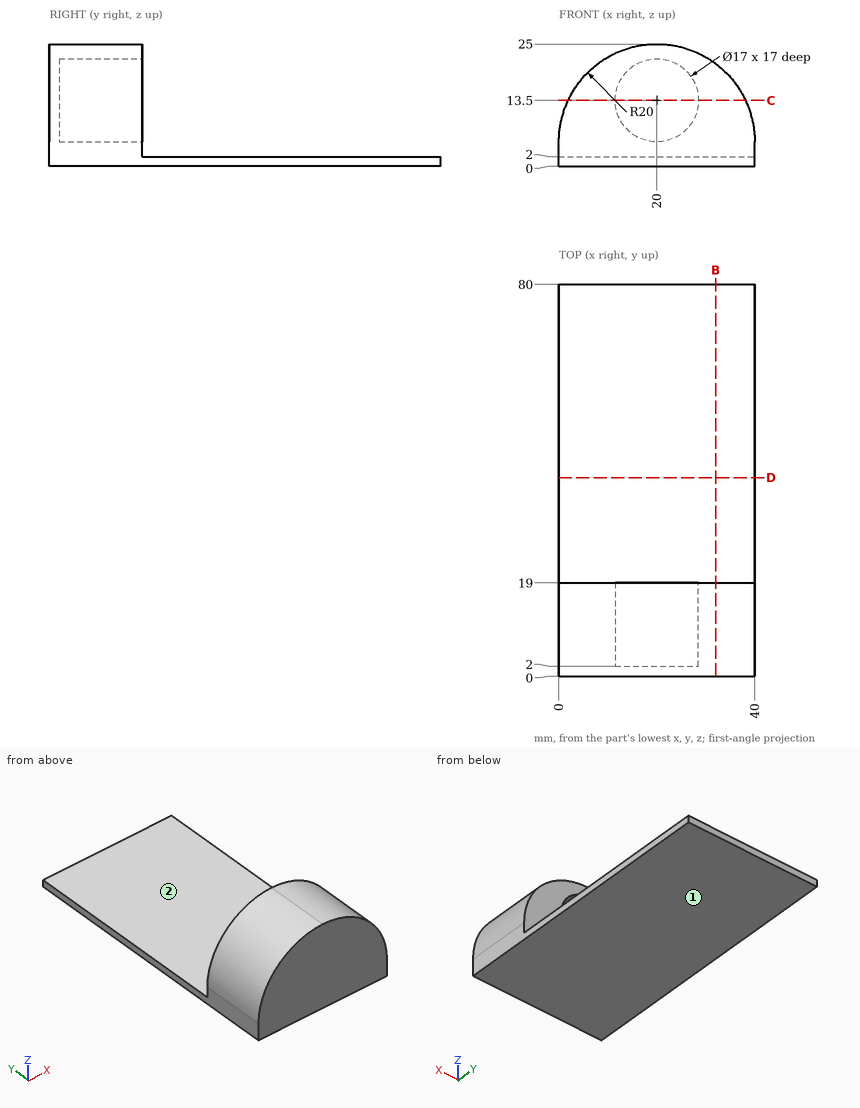
Check sheet for the drawn part. Datum: minimum x, y, z corner. Units: mm. A direction names the side the tool comes from. Give positions to 0.01 mm unless a question says otherwise; leave off trailing zeros. Write each loop counter-clockwise with the first axis right and the second up, starting at its lowest first coordinate (ties: lowest second). Pieces come first, ordered by that corner, then holes. Notation, with made-up numbers: M 66,-35 L 100,-35 A24 cw 100,-25 Z; hole C -39.75,-14.75 d2. An arc over 180 degrees is marked long. One line per question, with ' | ' between items.
1) Section check B-B on x = 32. Enter the section's corners in (y, z).
Result:
outline: M 0,0 L 80,0 L 80,2 L 19,2 L 19,21 L 0,21 Z
2) Section check D-D on y = 40.5. Enter the section's corners in (x, z).
Result:
outline: M 0,0 L 40,0 L 40,2 L 0,2 Z
3) Section check C-C on z = 13.5. Enter the section's corners in (x, y).
Result:
outline: M 1.9,0 L 38.1,0 L 38.1,19 L 28.5,19 L 28.5,2 L 11.5,2 L 11.5,19 L 1.9,19 Z
4) Thickness scan on line 1 along Z through (x, y) = (20, 15.5); line 2 along Z through (x, y) = (7, 71.5); line 3 along Y through (x, z) = (8, 11.5). Record the ranges inside material, lowest first. Write a range as [from, to].
Result:
line 1: z = [0, 5], [22, 25] | line 2: z = [0, 2] | line 3: y = [0, 19]
5) Set-up check for the marked faces 1 and 2: record each of +Z, -Z, +X, -X, +Y, -Y from which the full face is reachable in a straight line by a thin tool's end or side.
Result:
face 1: -Z, +X, -X, +Y, -Y | face 2: +Z, +X, -X, +Y
6) Gauge pin test, flat ends, axial feed: pin 1 Ø8 at (x, y) = (26, 60.5) entering from -Z; pin 2 Ø4 at (x, y) = (17.5, 43.5) entering from +Z; pin 3 Ø5 at (x, z) = (21, 17) entering from +Y; pin 4 Ø4 at (x, y) = (30, 18.5) entering from +Z. Record the tip position at first contact, or that the pin passes through.
Result:
pin 1: stops at z = 0 | pin 2: stops at z = 2 | pin 3: stops at y = 2 | pin 4: stops at z = 23.33
